The model under review builds one solid part; all positions refer to its coordinate system, in mm. A direction names the side the tool comes from. Coordinates: 2 decimals unless noted, no trailing zeros. Write each loop counter-clockwise with the first axis right and the second up, starting at its lowest first coordinate (ties: lowest second). Pieces come first, ordered by that corner, then holes. Notation, with made-up numbers: (24, 56.5) - (49, 56.5) arc R18 ccw to (49, 81.5) - close; hole circle Ø11 at (6.5, 38). An arc over 180 degrees is marked (long way). Answer as CSV lines item,"result". Start each with the question number.
```python
from build123d import *

# Parameters (mm, degrees)
BOSS_EXTRUDE1_DEPTH = 11
CUT_EXTRUDE1_DEPTH  = 9
SKETCH3_W           = 10
SKETCH3_H           = 1.5
CUT_EXTRUDE2_DEPTH  = 9
SKETCH4_W           = 10
SKETCH4_H           = 1.5
CUT_EXTRUDE3_DEPTH  = 9
SKETCH5_W           = 10
SKETCH5_H           = 1.5
CUT_EXTRUDE4_DEPTH  = 9
SKETCH6_R           = 1
CUT_EXTRUDE5_DEPTH  = 9
SKETCH7_R           = 1
CUT_EXTRUDE6_DEPTH  = 9
SKETCH8_R           = 1
CUT_EXTRUDE10_DEPTH = 9
BOSS_EXTRUDE2_DEPTH = 1
SKETCH11_W          = 0.5
SKETCH11_H          = 8
CUT_EXTRUDE12_DEPTH = 30.017236257
BOSS_EXTRUDE3_DEPTH = 2
SKETCH13_W          = 4
SKETCH13_H          = 8
BOSS_EXTRUDE4_DEPTH = 2
SKETCH14_R          = 1.5
CUT_EXTRUDE13_DEPTH = 10


with BuildPart() as part:
    # Sketch1 → Boss-Extrude1 (new body)
    with BuildSketch(Plane(origin=(0, 0, 0), x_dir=(1, 0, 0), z_dir=(0, 1, 0))):
        Polygon((-13.5, 0), (13.5, 0), (13.5, 8), (20, 8), (20, -19), (13.5, -19), (13.5, -5), (-13.5, -5), (-13.5, -19), (-20, -19), (-20, 8), (-13.5, 8), align=None)
    extrude(amount=BOSS_EXTRUDE1_DEPTH)

    # Sketch2 → Cut-Extrude1 (cut)
    with BuildSketch(Plane(origin=(0, 11, 0), x_dir=(1, 0, 0), z_dir=(0, 1, 0))):
        Polygon((-18, 8), (-18, -19), (-13.5, -19), (-13.5, -5), (13.5, -5), (13.5, -19), (18, -19), (18, 8), (13.5, 8), (13.5, -2), (-13.5, -2), (-13.5, 8), align=None)
    extrude(amount=-CUT_EXTRUDE1_DEPTH, mode=Mode.SUBTRACT)

    # Sketch3 → Cut-Extrude2 (cut)
    with BuildSketch(Plane.XY.offset(2)):
        with Locations((-8.5, 10.25)):
            Rectangle(SKETCH3_W, SKETCH3_H)
    extrude(amount=-CUT_EXTRUDE2_DEPTH, mode=Mode.SUBTRACT)

    # Sketch4 → Cut-Extrude3 (cut)
    with BuildSketch(Plane.ZY.offset(-18)):
        with Locations((-3, 10.25)):
            Rectangle(SKETCH4_W, SKETCH4_H)
    extrude(amount=-CUT_EXTRUDE3_DEPTH, mode=Mode.SUBTRACT)

    # Sketch5 → Cut-Extrude4 (cut)
    with BuildSketch(Plane(origin=(-18, 0, 0), x_dir=(0, 0, -1), z_dir=(1, 0, 0))):
        with Locations((-14, 10.25)):
            Rectangle(SKETCH5_W, SKETCH5_H)
    extrude(amount=-CUT_EXTRUDE4_DEPTH, mode=Mode.SUBTRACT)

    # Sketch6 → Cut-Extrude5 (cut)
    with BuildSketch(Plane(origin=(0, 0, 0), x_dir=(-1, 0, 0), z_dir=(0, 0, -1))):
        with Locations((11.75, 1.75)):
            Circle(SKETCH6_R)
        with Locations((-11.75, 9.25)):
            Circle(SKETCH6_R)
    extrude(amount=-CUT_EXTRUDE5_DEPTH, mode=Mode.SUBTRACT)

    # Sketch7 → Cut-Extrude6 (cut)
    with BuildSketch(Plane(origin=(20, 0, 0), x_dir=(0, 0, -1), z_dir=(1, 0, 0))):
        with Locations((6.25, 1.75)):
            Circle(SKETCH7_R)
        with Locations((-17.25, 9.25)):
            Circle(SKETCH7_R)
    extrude(amount=-CUT_EXTRUDE6_DEPTH, mode=Mode.SUBTRACT)

    # Sketch8 → Cut-Extrude10 (cut)
    with BuildSketch(Plane.ZY.offset(20)):
        with Locations((17.25, 1.75)):
            Circle(SKETCH8_R)
        with Locations((-6.25, 9.25)):
            Circle(SKETCH8_R)
    extrude(amount=-CUT_EXTRUDE10_DEPTH, mode=Mode.SUBTRACT)

    # Sketch10 → Boss-Extrude2 (add, symmetric)
    with BuildSketch(Plane(origin=(0, 0, 0), x_dir=(0, 0, -1), z_dir=(1, 0, 0))):
        Polygon((-5, 2), (-2, 2), (-2, 8.5), align=None)
    extrude(amount=BOSS_EXTRUDE2_DEPTH, both=True)

    # Sketch11 → Cut-Extrude12 (cut, through all)
    with BuildSketch(Plane(origin=(0, 2, 0), x_dir=(1, 0, 0), z_dir=(0, 1, 0))):
        with Locations((-13.75, 4)):
            Rectangle(SKETCH11_W, SKETCH11_H)
        with Locations((13.75, 4)):
            Rectangle(SKETCH11_W, SKETCH11_H)
    extrude(amount=-CUT_EXTRUDE12_DEPTH, mode=Mode.SUBTRACT)

    # Sketch12 → Boss-Extrude3 (add)
    with BuildSketch(Plane.XY.offset(2)):
        Polygon((-18, 8.5), (-15, 2), (-18, 2), align=None)
        Polygon((18, 2), (18, 8.5), (15, 2), align=None)
    extrude(amount=BOSS_EXTRUDE3_DEPTH)

    # Sketch13 → Boss-Extrude4 (add)
    with BuildSketch(Plane(origin=(0, 2, 0), x_dir=(1, 0, 0), z_dir=(0, 1, 0))):
        with Locations((11.5, -15)):
            Rectangle(SKETCH13_W, SKETCH13_H)
        with Locations((-11.5, -15)):
            Rectangle(SKETCH13_W, SKETCH13_H)
    extrude(amount=-BOSS_EXTRUDE4_DEPTH)

    # Sketch14 → Cut-Extrude13 (cut)
    with BuildSketch(Plane(origin=(0, 0, 0), x_dir=(-1, 0, 0), z_dir=(0, -1, 0))):
        with Locations(Location((-12, -14.174463975, 0), (0, 0, 90))):
            Circle(SKETCH14_R)
        with Locations(Location((12, -14.174463975, 0), (0, 0, 270))):
            Circle(SKETCH14_R)
    extrude(amount=-CUT_EXTRUDE13_DEPTH, mode=Mode.SUBTRACT)


solid = part.part
```
(1) Add section D-D on y = 4.25. Give the boundary of the cut face in (x, z), then the cut area to 3 significant figures.
(2) Add section B-B on z = -1.75. Give the boundary of the cut face in (x, y).
(3) Wall thickness on line 1 (X direction, y = 4.5, z = 17.75); line 2 (X direction, y = 3.75, z = 0.5); line 3 (Z direction, x = 16.9, y = 1.75): over which ranges is each line inside the solid? List them lowest first.
(4) Add section C-C on z = -6.25. Give the boundary of the cut face in (x, y), then the cut area to 3 significant figures.
(5) For pin 1 (3.5 mm diameter, centred on x = -17, y = 6, fed in from -Z); pin 2 (1.5 mm diameter, centred on x = 16, y = 5, fed in from -Z); pin 3 (6 mm diameter, centred on x = 10.5, z = 8.5, fed in from +Y); pin 4 (1 mm diameter, centred on x = 19.5, z = -3, fed in from +Y), all flat-tipped, find the tip position at first contact; note any pin that passes through.
(6) The part is to be moulded in two halves that separate along X. For faces 1 (the flat face through (18.3, 3.6, -8)), 2 (the cylindrical face through (11.88, 10.24, 0.99)), say which applies: released by +X, released by -X, zero draft, split by the parting line, or undercut.
(7) Add section A-A on z = 1. Give the boundary of the cut face in (x, y), then the cut area to 3 significant figures.
(8) For faces 3 (the flat face through (-9.5, 1, 15)), 4 (the flat face through (-14, 1, -4)), 5 (the flat face through (1, 4, 3)), 6 (the cylindrical face through (-17.518, 0.774, 17.033)), 7 (the flat face through (-16.521, 5.296, 2.986)), list the 3-axis set-ups (+Z, -Z, +X, -X, +Y, -Y) from which the entire face can be reached by the end or side of a thin tool; tool diameter is ignored.
Reported:
1,outline,"(-20, -8) - (-18, -8) - (-18, 2) - (-16.04, 2) - (-16.04, 4) - (-18, 4) - (-18, 19) - (-20, 19) - close; (-13.5, 0) - (13.5, 0) - (13.5, 2) - (1, 2) - (1, 3.96) - (-1, 3.96) - (-1, 2) - (-13.5, 2) - close; (16.04, 2) - (18, 2) - (18, -8) - (20, -8) - (20, 19) - (18, 19) - (18, 4) - (16.04, 4) - close"
1,area,"174 mm²"
2,outline,"(-20, 0) - (-14, 0) - (-14, 2) - (-18, 2) - (-18, 11) - (-20, 11) - close; (14, 0) - (20, 0) - (20, 9.5) - (18, 9.5) - (18, 2) - (14, 2) - close"
3,line 1,"-20 to -18, 18 to 20"
3,line 2,"-20 to -18, -13.5 to 13.5, 18 to 20"
3,line 3,"-8 to -7.25, -5.25 to 19"
4,outline,"(-20, 0) - (-14, 0) - (-14, 2) - (-18, 2) - (-18, 8.25) - (-20, 8.25) - close; (-20, 10.25) - (-18, 10.25) - (-18, 11) - (-20, 11) - close; (14, 0) - (20, 0) - (20, 0.75) - (14, 0.75) - close; (18, 2.75) - (20, 2.75) - (20, 9.5) - (18, 9.5) - close"
4,area,"44.0 mm²"
5,pin 1,"z = -8"
5,pin 2,"z = 2"
5,pin 3,"y = 2"
5,pin 4,"y = 9.5"
6,face 1,"zero draft"
6,face 2,"undercut"
7,outline,"(-20, 0) - (20, 0) - (20, 9.5) - (18, 9.5) - (18, 2) - (13.5, 2) - (13.5, 11) - (-3.5, 11) - (-3.5, 9.5) - (-13.5, 9.5) - (-13.5, 2) - (-18, 2) - (-18, 11) - (-20, 11) - close; hole circle Ø2 at (-11.75, 1.75); hole circle Ø2 at (11.75, 9.25)"
7,area,"335 mm²"
8,face 3,"+Z, +Y, -Y"
8,face 4,"-Z, +Y, -Y"
8,face 5,"+Z, +Y"
8,face 6,"-X"
8,face 7,"+Z, -Z, +Y"
